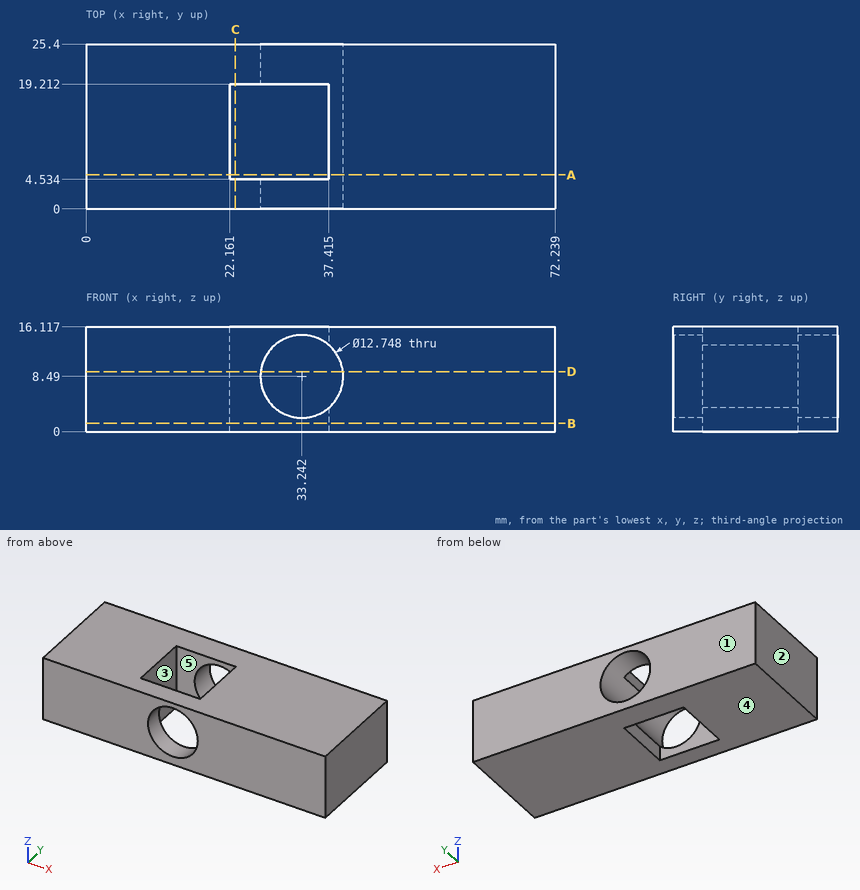
The drawing under review shows one solid part. Ordinate dimensions are in mm from its lowest x, y, z. A direction names the side the tool comes from. Round coordinates to 2 decimals unless told otherwise and drop trailing zeros. Order: outer loops, then holes, each group sorted by start corner. A loop starts at its lowest first (then second) coordinate and runs counter-clockwise, first axis right, second up. Notation, with made-up numbers: (6, 15) - (58, 15) arc R22 ccw to (58, 53) - close; hole circle Ø1 at (60, 69). An arc over 180 degrees is marked (long way). Return JSON: item names as keys, results as strings.
Q1. Consider section D-D on z = 9.25. Write out the cut boundary in (x, y), plus the area to 3 significant figures.
Computed values:
{"outline": "(0, 0) - (26.91, 0) - (26.91, 4.53) - (22.16, 4.53) - (22.16, 19.21) - (26.91, 19.21) - (26.91, 25.4) - (0, 25.4) - close; (39.57, 0) - (72.24, 0) - (72.24, 25.4) - (39.57, 25.4) - close", "area": "1,440 mm2"}
Q2. The part is to be moulded in two halves that separate along X. For the marked faces 1, 2 and 3, say which applies: pulls with the +X half, pulls with the -X half, needs draft (parallel to the pull), parting line crosses it, or undercut.
Computed values:
{"face 1": "needs draft", "face 2": "pulls with the -X half", "face 3": "undercut"}
Q3. Machinability: for the marked faces 4 and 5, which of the approach directions +Z, -Z, +X, -X, +Y, -Y give a long, thin tool a straight path to every point of the face, cutting with its end or side? Answer none if there is none.
Computed values:
{"face 4": "-Z, +X, -X, +Y, -Y", "face 5": "+Z, -Z"}
Q4. For pin 1 Ø4.5 at (x, z) = (31, 7.5) entering from -Y, flat-tipped, find the tip position at first contact; note if it passes through.
Computed values:
{"pin 1": "passes through"}
Q5. Wall thickness on L1, parallel to Y at x = 32.5, z = 15; L2, parallel to X at y = 11, z = 15 (1 decimal); L3, parallel to X at y = 24, z = 8.5 (1 decimal): over which ranges is each line inside the solid? List them lowest first. Write a range as [from, to].
Computed values:
{"L1": "y = [0, 4.53], [19.21, 25.4]", "L2": "x = [0, 22.2], [37.4, 72.2]", "L3": "x = [0, 26.9], [39.6, 72.2]"}
Q6. Consider section A-A on y = 5.25. Write out the cut boundary in (x, z) (1 decimal), plus the area to 3 significant figures.
Computed values:
{"outline": "(0, 0) - (22.2, 0) - (22.2, 16.1) - (0, 16.1) - close; (37.4, 0) - (72.2, 0) - (72.2, 16.1) - (37.4, 16.1) - (37.4, 13.3) arc R6.4 cw to (37.4, 3.7) - close", "area": "904 mm2"}
Q7. Consider section C-C on x = 23. Write out the cut boundary in (y, z), plus the area to 3 significant figures.
Computed values:
{"outline": "(0, 0) - (4.53, 0) - (4.53, 16.12) - (0, 16.12) - close; (19.21, 0) - (25.4, 0) - (25.4, 16.12) - (19.21, 16.12) - close", "area": "173 mm2"}
Q8. Consider section B-B on z = 1.25. Write out the cut boundary in (x, y) (1 decimal).
Computed values:
{"outline": "(0, 0) - (72.2, 0) - (72.2, 25.4) - (0, 25.4) - close; hole (22.2, 4.5) - (37.4, 4.5) - (37.4, 19.2) - (22.2, 19.2) - close"}
